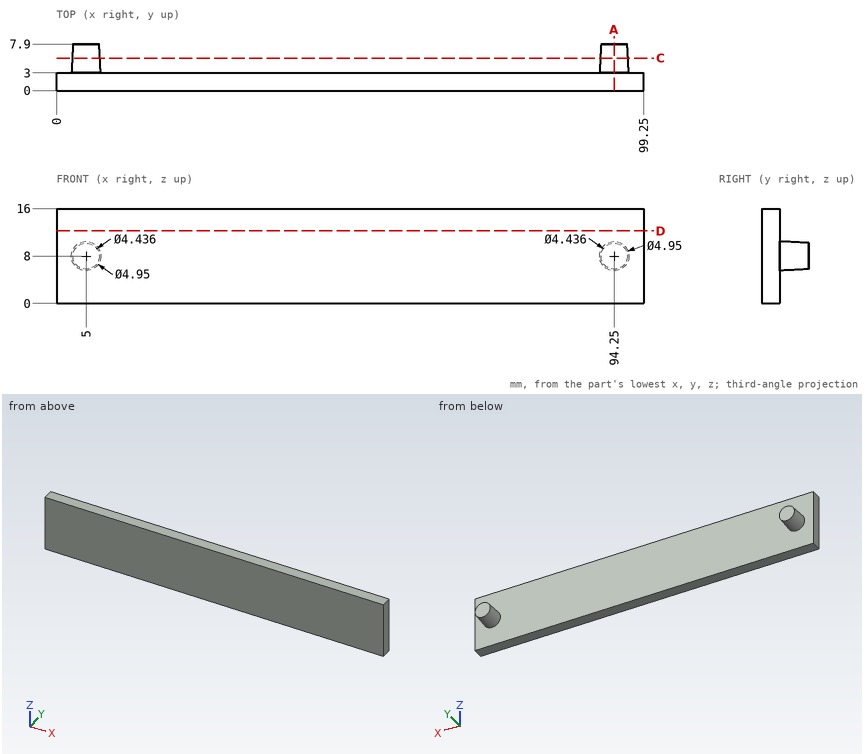
The figure shows three views and two pictorial views of one solid part (mm, origin at its lowest corner). Answer the questions. Coordinates: 2 decimals unless noted, no trailing zeros. Loops run counter-clockwise (first coordinate to the right, second up) from the corner with the lowest first, then second, coordinate; pieces in that order, holes last. Notation, with made-up numbers: M 52.5,11.25 L 82.5,11.25 A14 ccw 82.5,15.25 Z; hole C 7,-28 d11. An arc over 180 degrees is marked long. Use CSV: the item, a comma, the result in double quotes. Start each with the question number.
(1) Consider line 1 (X direction, y = 4, z = 7) (1 decimal); line 2 (Y direction, x = 81, z = 14); line 3 (X direction, y = 6, z = 8.75). Determine where each line is inside the solid, lowest interval first.
(2) Find section D-D, the plane z = 12.25. Give the vertices of the cut face in (x, y), then the cut area to 3 significant figures.
(3) Given pin 1 Ø2 at (x, z) = (16, 13.5) entering from +Y; pin 2 Ø4 at (y, z) = (4, 3) entering from +X, each flat-ended and moving along its own axis, determine where each tip first touches the part or whether it passes through.
(4) Find section C-C, the plane y = 5.5. Give the vertices of the cut face in (x, z).
(5) Find section A-A, the plane x = 94.25. Give the vertices of the cut face in (y, z) (1 decimal), then the cut area to 3 significant figures.
Recorded:
1,line 1,"x = 2.8 to 7.2, 92 to 96.5"
1,line 2,"y = 0 to 3"
1,line 3,"x = 2.81 to 7.19, 92.06 to 96.44"
2,outline,"M 0,0 L 99.25,0 L 99.25,3 L 0,3 Z"
2,area,"298 mm^2"
3,pin 1,"stops at y = 3"
3,pin 2,"stops at x = 99.25"
4,outline,"C 5,8 d4.69; C 94.25,8 d4.69"
5,outline,"M 0,0 L 3,0 L 3,5.5 L 7.9,5.8 L 7.9,10.2 L 3,10.5 L 3,16 L 0,16 Z"
5,area,"71.0 mm^2"
